from build123d import *

# Parameters (mm, degrees)
BOSS_EXTRUDE1_DEPTH = 20
SKETCH2_R           = 10
CUT_EXTRUDE1_DEPTH  = 20
LPATTERN1_COUNT     = 3
LPATTERN1_PITCH     = 90
SKETCH4_R           = 10
CUT_EXTRUDE2_DEPTH  = 20
LPATTERN2_COUNT     = 3
LPATTERN2_PITCH     = 90
SKETCH5_R           = 7.5
CUT_EXTRUDE4_DEPTH  = 20
LPATTERN4_COUNT     = 3
LPATTERN4_PITCH     = 90
BOSS_EXTRUDE3_DEPTH = 60


with BuildPart() as part:
    # Sketch1 → Boss-Extrude1 (new body)
    with BuildSketch(Plane(origin=(0, 0, 0), x_dir=(1, 0, 0), z_dir=(0, 1, 0))):
        with BuildLine():
            Line((-90, -75), (90, -75))
            ThreePointArc((90, -75), (165, 0), (90, 75))
            Line((90, 75), (-90, 75))
            ThreePointArc((-90, 75), (-165, 0), (-90, -75))
        make_face()
    extrude(amount=BOSS_EXTRUDE1_DEPTH)

    # Sketch2 → Cut-Extrude1 (cut)
    with BuildSketch(Plane(origin=(0, 20, 0), x_dir=(1, 0, 0), z_dir=(0, 1, 0))):
        with Locations((-90, 55)):
            Circle(SKETCH2_R)
    cut_extrude1 = extrude(amount=-CUT_EXTRUDE1_DEPTH, mode=Mode.SUBTRACT)

    # LPattern1: Cut-Extrude1 ×3
    with Locations(*[(i * LPATTERN1_PITCH, 0, 0) for i in range(1, LPATTERN1_COUNT)]):
        add(cut_extrude1, mode=Mode.SUBTRACT)

    # Sketch4 → Cut-Extrude2 (cut)
    with BuildSketch(Plane(origin=(0, 20, 0), x_dir=(1, 0, 0), z_dir=(0, 1, 0))):
        with Locations((-90, -55)):
            Circle(SKETCH4_R)
    cut_extrude2 = extrude(amount=-CUT_EXTRUDE2_DEPTH, mode=Mode.SUBTRACT)

    # LPattern2: Cut-Extrude2 ×3
    with Locations(*[(i * LPATTERN2_PITCH, 0, 0) for i in range(1, LPATTERN2_COUNT)]):
        add(cut_extrude2, mode=Mode.SUBTRACT)

    # Sketch5 → Cut-Extrude4 (cut)
    with BuildSketch(Plane(origin=(0, 20, 0), x_dir=(1, 0, 0), z_dir=(0, 1, 0))):
        with Locations((-90, 0)):
            Circle(SKETCH5_R)
    cut_extrude4 = extrude(amount=-CUT_EXTRUDE4_DEPTH, mode=Mode.SUBTRACT)

    # LPattern4: Cut-Extrude4 ×3
    with Locations(*[(i * LPATTERN4_PITCH, 0, 0) for i in range(1, LPATTERN4_COUNT)]):
        add(cut_extrude4, mode=Mode.SUBTRACT)

    # Sketch6 → Boss-Extrude3 (add)
    with BuildSketch(Plane(origin=(0, 20, 0), x_dir=(1, 0, 0), z_dir=(0, 1, 0))):
        with BuildLine():
            Line((-90, 36.456417916), (90, 36.456417916))
            ThreePointArc((90, 36.456417916), (126.456417916, 0), (90, -36.456417916))
            Line((90, -36.456417916), (-90, -36.456417916))
            ThreePointArc((-90, -36.456417916), (-126.456417916, 0), (-90, 36.456417916))
        make_face()
        with BuildLine():
            Line((-90, 25.16029231), (90, 25.16029231))
            ThreePointArc((90, 25.16029231), (115.16029231, 0), (90, -25.16029231))
            Line((90, -25.16029231), (-90, -25.16029231))
            ThreePointArc((-90, -25.16029231), (-115.16029231, 0), (-90, 25.16029231))
        make_face(mode=Mode.SUBTRACT)
    extrude(amount=BOSS_EXTRUDE3_DEPTH)


solid = part.part
Source: CAD feature listing. Evaluate the final solid. Frame: model axes, mm. A direction names the side the tool comes from. Give positions to 0.01 mm unless a question says otherwise; leave off trailing zeros. Write each loop counter-clockwise with the first axis right and the second up, starting at its lowest first coordinate (ties: lowest second). Pieces come first, ordered by that corner, then holes. Notation, with made-up numbers: M -38,-34 L 2,-34 A37 ccw 2,4 Z; hole C 43.25,-26.5 d7. An arc over 180 degrees is marked long. Answer as a JSON object with one key per item and string values.
Q1. Cut plane D-D, the plane z = -13. Return the cut outline in (x, y), then the cut area to 3 significant figures.
Geometry check:
{"outline": "M -163.86,0 L 163.86,0 L 163.86,20 L 124.06,20 L 124.06,80 L 111.54,80 L 111.54,20 L -111.54,20 L -111.54,80 L -124.06,80 L -124.06,20 L -163.86,20 Z", "area": "8,060 mm^2"}
Q2. Cut plane B-B, the plane x = 0. Return the cut outline in (y, z), then the cut area to 3 significant figures.
Geometry check:
{"outline": "M 0,-75 L 20,-75 L 20,-65 L 0,-65 Z; M 0,-45 L 20,-45 L 20,-36.46 L 80,-36.46 L 80,-25.16 L 20,-25.16 L 20,-7.5 L 0,-7.5 Z; M 0,7.5 L 20,7.5 L 20,25.16 L 80,25.16 L 80,36.46 L 20,36.46 L 20,45 L 0,45 Z; M 0,65 L 20,65 L 20,75 L 0,75 Z", "area": "3,260 mm^2"}
Q3. Contact query for flat-ended pins moving along their axis: P1, Ø13.5, axis at x = -90, z = 0, coming from the -Y side; P2, Ø6, axis at y = 27, z = -17, coming from the -X side; P3, Ø5, axis at x = -122, y = 36.5, coming from the -Z side; P4, Ø1.5, axis at x = -48, y = 71.5, coming from the -Z side. Output: stop coordinate, or through.
Geometry check:
{"P1": "passes through", "P2": "stops at x = -123.66", "P3": "stops at z = -21.42", "P4": "stops at z = -36.46"}
Q4. Ray query, line 1 along Z through (x, y) = (0, 4.5); line 2 along X through (y, z) = (15.25, 0); line 3 along Z through (x, y) = (34.5, 67.5). Return the intervals inside material, ascending.
Geometry check:
{"line 1": "z = -75 to -65, -45 to -7.5, 7.5 to 45, 65 to 75", "line 2": "x = -165 to -97.5, -82.5 to -7.5, 7.5 to 82.5, 97.5 to 165", "line 3": "z = -36.46 to -25.16, 25.16 to 36.46"}
Q5. Mould query, pull axis Z, two halves, no side actions, for faces 5 (the face through (1, 10, -75)), 6 (the face through (82, 10, -49)), 7 (the face through (-1, 10, 75)). Classes: +Z half, -Z half, draft (parallel to the pull), parting line (faces both ways), or undercut.
Geometry check:
{"face 5": "-Z half", "face 6": "undercut", "face 7": "+Z half"}
Q6. Access query for faces 1 (the face through (-126.448, 49.58, 0.802)), 2 (the face through (-2, 0, -18)), 3 (the face through (1, 50, 36.456)), 4 (the face through (115.154, 49.58, -0.553)). Directions: +Z, -Z, +X, -X, +Y, -Y. A direction counts if a zero-diameter tool reaches every point of the face in a straight line with its end or side. Return the directions, or none.
Geometry check:
{"face 1": "-X, +Y", "face 2": "+Z, -Z, +X, -X, -Y", "face 3": "+Z, +X, -X, +Y", "face 4": "+Y"}
Q7. Cut plane C-C, the plane z = 55. Return the cut outline in (x, y).
Geometry check:
{"outline": "M -140.99,0 L -100,0 L -100,20 L -140.99,20 Z; M -80,0 L -10,0 L -10,20 L -80,20 Z; M 10,0 L 80,0 L 80,20 L 10,20 Z; M 100,0 L 140.99,0 L 140.99,20 L 100,20 Z"}
Q8. Cut plane A-A, the plane y = 56. Return the cut outline in (x, z).
Geometry check:
{"outline": "M -90,-36.46 L 90,-36.46 A36.46 ccw 90,36.46 L -90,36.46 A36.46 ccw Z; hole M -90,-25.16 L 90,-25.16 A25.16 ccw 90,25.16 L -90,25.16 A25.16 ccw Z"}
